Geometry check sheet. Reference: the model listing, model coordinates, mm. A direction names the side the tool comes from. Coordinates: 2 decimals unless noted, no trailing zeros. Order: outer loops, then holes, each group sorted by start corner. A loop starts at its lowest first (then second) coordinate and runs counter-clockwise, first axis right, second up. Notation, with made-up numbers: (40.5, -31) - (48.5, -31) arc R21 ccw to (48.5, 6) - close; hole circle Ø9 at (-28.5, 42). An arc over 180 degrees is marked (long way). One line per item, written item: value. Start each with the question number.
```python
from build123d import *

# Parameters (mm, degrees)
CUT_EXTRUDE1_DEPTH      = 2
CUT_EXTRUDE1_DEPTH_BACK = 2


with BuildPart() as part:
    # Sketch1 → Revolve1 (revolve)
    with BuildSketch(Plane.XY, mode=Mode.PRIVATE) as revolve1_sk:
        Polygon((-4, 0), (-4, 3.5), (0, 3.5), (0, 2.35), (0.6, 2), (15.5705, 2), (16, 1.5705), (16, 0), align=None)
    revolve(revolve1_sk.sketch.rotate(Axis((16, 0, 0), (-1, 0, 0)), 270), axis=Axis((16, 0, 0), (-1, 0, 0)))

    # Sketch2 → Cut-Revolve1 (revolve, cut)
    with BuildSketch(Plane.XY, mode=Mode.PRIVATE) as cut_revolve1_sk:
        Polygon((-4, 3.1), (-3.6, 3.5), (-0.235, 3.5), (0, 3.265), (0, 4.2), (-4, 4.2), align=None)
    revolve(cut_revolve1_sk.sketch.rotate(Axis((0, 0, 0), (-1, 0, 0)), 270), axis=Axis((0, 0, 0), (-1, 0, 0)), mode=Mode.SUBTRACT)

    # Sketch3 → Cut-Revolve2 (revolve, cut)
    with BuildSketch(Plane.XY, mode=Mode.PRIVATE) as cut_revolve2_sk:
        Polygon((-4, 0), (-4, 1.71), (-3.79, 1.5), (-2, 1.5), (-1.133974596, 0), align=None)
    revolve(cut_revolve2_sk.sketch.rotate(Axis((-1.133974596, 0, 0), (-1, 0, 0)), 270), axis=Axis((-1.133974596, 0, 0), (-1, 0, 0)), mode=Mode.SUBTRACT)

    # Sketch4 → Cut-Extrude1 (cut, two sides: drawn at the far end of the back side and taken through both)
    with BuildSketch(Plane(origin=(-4, 0, 0), x_dir=(0, 0, -1), z_dir=(1, 0, 0)).offset(-CUT_EXTRUDE1_DEPTH_BACK)):
        Polygon((-1.5, -0.866025404), (0, -1.732050808), (1.5, -0.866025404), (1.5, 0.866025404), (0, 1.732050808), (-1.5, 0.866025404), align=None)
    extrude(amount=CUT_EXTRUDE1_DEPTH + CUT_EXTRUDE1_DEPTH_BACK, mode=Mode.SUBTRACT)


solid = part.part
```
Q1. Release check for a two-part mould opening along Y. For faces 1 (the cylindrical face through (8, -2, 0)), 2 (the flat face through (16, 0, 0)), 3 (the flat face through (-3.014, 1.305, 0.74)), 4 (the flat face through (-3.014, 1.293, -0.76)) record: released by +Y, released by -Y, zero draft, split by the parting line, or undercut.
Q2. Set-up check for faces 5 (the flat face through (-3, 0, -1.5)), 6 (the flat face through (-4, -1.33, -1.33)), 7 (the flat face through (0, -1.4, 2.1)): record each of +Z, -Z, +X, -X, +Y, -Y from which the full face is reachable in a straight line by a thin tool's end or side.
Q3. Material ranges on probe 1 along X at (y, z) = (-2.5, -1); probe 2 along Y at (x, z) = (12.5, 0); probe 3 along X at (y, z) = (3.25, 1), recorded low to high.
Q4. Gauge pin test, flat ends, axial feed: P1, Ø2, axis at x = 7, y = 0, coming from the +Z side; P2, Ø4, axis at y = -2, z = -2.5, coming from the +X side; P3, Ø1.5, axis at x = 12, z = -1, coming from the -Y side. Record the tip position at first contact, or that the pin passes through.
Q5. Cross-section at A-A, the plane x = 8. Enter the section's corners in (y, z).
Check result:
1. face 1: split by the parting line
1. face 2: zero draft
1. face 3: undercut
1. face 4: undercut
2. face 5: -X
2. face 6: +Z, -Z, -X, +Y, -Y
2. face 7: +X
3. probe 1: x = -4 to 0
3. probe 2: y = -2 to 2
3. probe 3: x = -3.7 to -0.14
4. P1: stops at z = 2
4. P2: stops at x = 16
4. P3: stops at y = -1.98
5. outline: circle Ø4 at (0, 0)
